Model file for the job. Use its own axes, mm. Face numbers are marked on the shaded views. A direction names the side the tool comes from. Round coordinates to 2 decimals unless told otherwise and drop trailing zeros. Loops run counter-clockwise (first coordinate to the right, second up) from the corner with the lowest first, then second, coordinate; pieces in that order, holes last. Notation, with made-up numbers: M 81,50.5 L 94,50.5 A35 cw 94,83.5 Z; hole C 46,7.25 d10. An arc over 180 degrees is marked long. Use a Markdown table: item, result. Add a question column.
Q1. Mould opens along Y. For the marked faces 4, 5, 6 and 7 say: +Y half, -Y half, draft (parallel to the pull), parting line (faces both ways), or undercut.
Q2. Tool access for the marked faces 1, 2 and 3: list every direction of +Z, -Z, +X, -X, +Y, -Y with a clear straight run to the whole face (end or side of a thin tool).
Q3. Cut at B-B (y = 7.5). Give the cut face in (x, z), plus the area to 3 significant figures.
Q4. Probe line 1 (Y direction, x = -28, z = 6.75); line 2 (X direction, y = -14.5, z = 15.5); line 3 (X direction, y = -3.5, z = 3.75). List the from-to ranges inside material, lowest first. Write a range as from..to.
Q5. Cut at D-D (x = 32.5). Give the cut face in (y, z), plus the area to 3 significant figures.
Q6. Pin check, flat tips, straight feed: pin 1 (3 mm diameter, centred on x = 33.5, y = -4.5, fed in from +Z); pin 2 (10 mm diameter, centred on y = 3.5, z = 15.5, fed in from +X); pin 3 (6 mm diameter, centred on x = -15, z = 14, fed in from +Y); pin 4 (1.5 mm diameter, centred on y = 24, z = 5, fed in from +X). Stop position of each tip, or through.
Q7. Cut at C-C (x = -19). Give the cut face in (y, z).
Q8. Cut at A-A (z = 17). Give the cut face in (x, y).
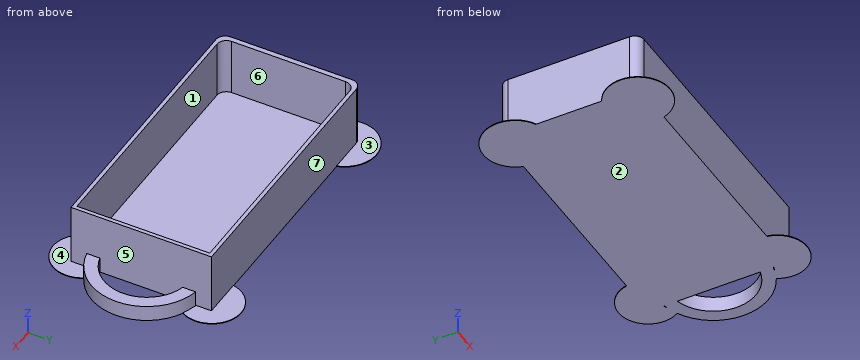
from build123d import *

# Parameters (mm, degrees)
SKETCH_1_W          = 86
SKETCH_1_H          = 44.4
EXTRUDE_1_DEPTH     = 19.6
EXTRUDE_2_DEPTH     = 5
SKETCH_3_W          = 83.2
SKETCH_3_H          = 42
CUT_EXTRUDE_1_DEPTH = 18.4
FILLET_1_R          = 3
EXTRUDE_3_DEPTH     = 0.2


with BuildPart() as part:
    # Эскиз1 → Бобышка-Вытянуть1 (new body)
    with BuildSketch(Plane.XY):
        Rectangle(SKETCH_1_W, SKETCH_1_H)
    extrude(amount=EXTRUDE_1_DEPTH)

    # Эскиз2 → Бобышка-Вытянуть2 (add)
    with BuildSketch(Plane.XY):
        with BuildLine():
            Line((43, 17.2), (43, 13.108775687))
            ThreePointArc((43, 13.108775687), (53.273546839, 0), (43, -13.108775687))
            Line((43, -13.108775687), (43, -17.2))
            ThreePointArc((43, -17.2), (57.273546839, 0), (43, 17.2))
        make_face()
    extrude(amount=EXTRUDE_2_DEPTH)

    # Эскиз3 → Вырез-Вытянуть1 (cut)
    with BuildSketch(Plane.XY.offset(19.6)):
        with Locations((0.2, 0)):
            Rectangle(SKETCH_3_W, SKETCH_3_H)
    extrude(amount=-CUT_EXTRUDE_1_DEPTH, mode=Mode.SUBTRACT)

    # Скругление1
    fillet_1_edges = [part.edges().sort_by_distance(p)[0] for p in [
        (-41.4, -21, 10.4),
        (-41.4, 21, 10.4),
        (-43, -22.2, 9.8),
        (-43, 22.2, 9.8),
    ]]
    fillet(fillet_1_edges, radius=FILLET_1_R)

    # Эскиз4 → Бобышка-Вытянуть3 (add)
    with BuildSketch(Plane(origin=(0, 0, 0), x_dir=(-1, 0, 0), z_dir=(0, 0, -1))):
        with BuildLine():
            Line((-47.582884167, 15.66091474), (-30.44547065, 22.2))
            ThreePointArc((-30.44547065, 22.2), (-42.919306358, 29.16488726), (-47.582884167, 15.66091474))
        make_face()
        with BuildLine():
            Line((-47.582884167, -15.66091474), (-30.44547065, -22.2))
            ThreePointArc((-30.44547065, -22.2), (-42.919306358, -29.16488726), (-47.582884167, -15.66091474))
        make_face()
        with BuildLine():
            Line((43, 10.417706136), (28.64602487, 22.2))
            ThreePointArc((28.64602487, 22.2), (44.771493482, 27.210488681), (43, 10.417706136))
        make_face()
        with BuildLine():
            Line((43, -10.417706136), (28.64602487, -22.2))
            ThreePointArc((28.64602487, -22.2), (44.771493482, -27.210488681), (43, -10.417706136))
        make_face()
    extrude(amount=-EXTRUDE_3_DEPTH)


solid = part.part
Checked values:
| question | item | result |
|---|---|---|
| 1 | face 4 | draft |
| 1 | face 5 | undercut |
| 1 | face 6 | undercut |
| 1 | face 7 | +Y half |
| 2 | face 1 | +Z |
| 2 | face 2 | -Z, +X, -X, +Y, -Y |
| 2 | face 3 | +Z, -X, +Y |
| 3 | outline | M -43,0 L 43,0 L 43,19.6 L 41.8,19.6 L 41.8,1.2 L -41.4,1.2 L -41.4,19.6 L -43,19.6 Z; M 51,0 L 55.58,0 L 55.58,5 L 51,5 Z |
| 3 | area | 178 mm^2 |
| 4 | line 1 | y = -22.2..-21, 21..22.2 |
| 4 | line 2 | x = -43..-41.4, 41.8..43 |
| 4 | line 3 | x = -43..-41.4, 41.8..43, 52.81..56.92 |
| 5 | outline | M -26.49,0 L 26.49,0 L 26.49,0.2 L 22.2,0.2 L 22.2,19.6 L 21,19.6 L 21,1.2 L -21,1.2 L -21,19.6 L -22.2,19.6 L -22.2,0.2 L -26.49,0.2 Z |
| 5 | area | 99.2 mm^2 |
| 6 | pin 1 | stops at z = 1.2 |
| 6 | pin 2 | stops at x = 43 |
| 6 | pin 3 | stops at y = 22.2 |
| 6 | pin 4 | passes through |
| 7 | outline | M -22.2,0 L 22.2,0 L 22.2,19.6 L 21,19.6 L 21,1.2 L -21,1.2 L -21,19.6 L -22.2,19.6 Z |
| 8 | outline | M -43,-19.2 A3 ccw -40,-22.2 L 43,-22.2 L 43,22.2 L -40,22.2 A3 ccw -43,19.2 Z; hole M -41.4,-18 A3 ccw -38.4,-21 L 41.8,-21 L 41.8,21 L -38.4,21 A3 ccw -41.4,18 Z |
